Input: part model. Units: mm. Frame: model coordinates. Face numbers are marked on the shaded views. Round coordinates to 2 decimals unless told otherwise and drop trailing zeros. Order: outer loops, then holes, each group sorted by start corner. A loop starts at its lowest first (then second) coordinate and runs counter-clockwise, first axis right, second up.
Item 1: First-contact query: pin 1 (1.6 mm diameter, centred on x = 41.25, z = 0, fed in from +Y); pin 2 (3 mm diameter, centred on y = 1.5, z = 29.5, fed in from +X); pin 3 (1.5 mm diameter, centred on y = 5.5, z = -7.5, fed in from -X); pin 4 (1.5 mm diameter, centred on x = -29, y = 7, fed in from -Z). Flat tips, straight axial feed; report the tip coordinate or a pass-through.
Item 2: Cut plane A-A on y = 6.25. Output: boundary loops of the cut face in (x, z).
Item 3: Cut plane B-B on z = 14. Output: boundary loops of the cut face in (x, y).
Item 4: Line query: L1, parallel to X at y = 5.75, z = 0; L2, parallel to Z at x = 41.25, y = 6; L3, parallel to X at y = 6.5, z = -8. Output: solid intervals per line, ascending.
Item 5: Cut plane C-C on x = -29.5. Output: boundary loops of the cut face in (y, z).
Item 6: Mould query, pull axis X, two halves, no side actions, for the marked faces 1, 2, 3 and 4. Classes: released by +X, released by -X, zero draft, split by the parting line, or undercut.
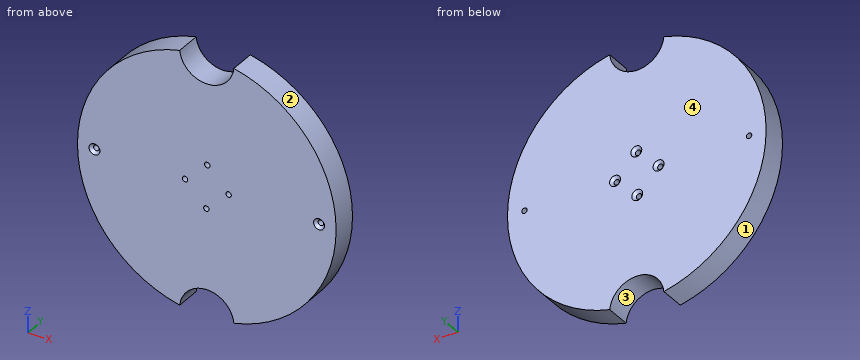
```python
from build123d import *

# Parameters (mm, degrees)
SKETCH1_R                = 47.5
BOSS_EXTRUDE1_DEPTH      = 9.5
CUT_EXTRUDE1_DEPTH       = 9.5
CAVITY1_OUTLINE_R        = 1
CAVITY1_DEPTH            = 9.5
CHAMFER1_SIZE            = 1
SKETCH3_R                = 1
CUT_EXTRUDE2_DEPTH       = 9.5
CHAMFER2_SIZE            = 1
CHAMFER2_OF_MIRROR2_SIZE = 1


# Read off the part's stored shape, not the designer's step: Cavity1
with BuildPart() as part:
    # Sketch1 → Boss-Extrude1 (new body)
    with BuildSketch(Plane(origin=(0, 0, 0), x_dir=(1, 0, 0), z_dir=(0, 1, 0))):
        with Locations(Location((0, 0, 0), (0, 0, 270))):
            Circle(SKETCH1_R)
    extrude(amount=BOSS_EXTRUDE1_DEPTH)

    # Sketch2 → Cut-Extrude1 (cut)
    with BuildSketch(Plane(origin=(0, 9.5, 0), x_dir=(1, 0, 0), z_dir=(0, 1, 0))):
        with BuildLine():
            Line((-10, 47.5), (10, 47.5))
            ThreePointArc((10, 47.5), (0, 37.5), (-10, 47.5))
        make_face()
    cut_extrude1 = extrude(amount=-CUT_EXTRUDE1_DEPTH, mode=Mode.SUBTRACT)

    # Mirror1: Cut-Extrude1 across plane
    add(cut_extrude1.mirror(Plane.XY), mode=Mode.SUBTRACT)

    # Cavity1 outline → Cavity1 (cut)
    with BuildSketch(Plane(origin=(0, 0, 0), x_dir=(1, 0, 0), z_dir=(0, 1, 0))):
        with Locations((7.9981372, 0.17263061)):
            Circle(CAVITY1_OUTLINE_R)
        with Locations((0.17263061, -7.9981372)):
            Circle(CAVITY1_OUTLINE_R)
        with Locations((-0.17263061, 7.9981372)):
            Circle(CAVITY1_OUTLINE_R)
        with Locations((-7.9981372, -0.17263061)):
            Circle(CAVITY1_OUTLINE_R)
    extrude(amount=CAVITY1_DEPTH, mode=Mode.SUBTRACT)

    # Chamfer1
    chamfer1_edges = [part.edges().sort_by_distance(p)[0] for p in [
        (-8.9981372, 9.5, 0.17263061),
        (-1.17263061, 9.5, -7.9981372),
        (-0.82736939, 9.5, 7.9981372),
        (6.9981372, 9.5, -0.17263061),
    ]]
    chamfer(chamfer1_edges, length=CHAMFER1_SIZE)

    # Sketch3 → Cut-Extrude2 (cut)
    with BuildSketch(Plane(origin=(0, 9.5, 0), x_dir=(1, 0, 0), z_dir=(0, 1, 0))):
        with Locations(Location((-41.25, 0, 0), (0, 0, 270))):
            Circle(SKETCH3_R)
    cut_extrude2 = extrude(amount=-CUT_EXTRUDE2_DEPTH, mode=Mode.SUBTRACT)

    # Chamfer2
    chamfer2_edges = [part.edges().sort_by_distance(p)[0] for p in [
        (-41.25, 0, -1),
    ]]
    chamfer(chamfer2_edges, length=CHAMFER2_SIZE)

    # Mirror2: Cut-Extrude2 across plane
    add(cut_extrude2.mirror(Plane(origin=(0, 0, 0), x_dir=(0, 0, 1), z_dir=(1, 0, 0))), mode=Mode.SUBTRACT)

    # Chamfer2 of Mirror2
    chamfer2_of_mirror2_edges = [part.edges().sort_by_distance(p)[0] for p in [
        (41.25, 0, -1),
    ]]
    chamfer(chamfer2_of_mirror2_edges, length=CHAMFER2_OF_MIRROR2_SIZE)


solid = part.part
```
From the geometry:
1. pin 1: passes through
1. pin 2: stops at x = 38.37
1. pin 3: stops at x = -47.02
1. pin 4: stops at z = -38.19
2. outline: (-9.94, -46.45) arc R10 cw to (9.94, -46.45) arc R47.5 ccw to (9.94, 46.45) arc R10 cw to (-9.94, 46.45) arc R47.5 ccw to start; hole circle Ø2 at (-41.25, 0); hole circle Ø2 at (-8, 0.17); hole circle Ø2 at (-0.17, -8); hole circle Ø2 at (0.17, 8); hole circle Ø2 at (8, -0.17); hole circle Ø2 at (41.25, 0)
3. outline: (-45.39, 0) - (45.39, 0) - (45.39, 9.5) - (-45.39, 9.5) - close
4. L1: x = -47.5 to -42.25, -40.25 to -8.98, -7.01 to 7.01, 8.98 to 40.25, 42.25 to 47.5
4. L2: z = -23.55 to -1, 1 to 23.55
4. L3: x = -46.82 to -1.17, 0.83 to 46.82
5. outline: (0, -37.23) - (9.5, -37.23) - (9.5, 37.23) - (0, 37.23) - close
6. face 1: released by -X
6. face 2: released by +X
6. face 3: undercut
6. face 4: zero draft
